Autodesk Inventor part; units mm, degrees
ref_plane "YZ Plane" through (0, 0, 0) normal (1, 0, 0) x (0, 1, 0)
ref_plane "XZ Plane" through (0, 0, 0) normal (0, 1, 0) x (-1, 0, 0)
ref_plane "XY Plane" through (0, 0, 0) normal (0, 0, 1) x (1, 0, 0)
sketch "草圖1" plane through (0, 0, 0) normal (0, 1, 0) x (-1, 0, 0)
  circle A0 centre (0, 0) radius 30
  line L0 (0, -30) -> (-70, -30)
  arc A1 (-70, 30) -> (-70, -30) centre (-70, 0) ccw
  line L1 (0, 30) -> (-70, 30)
  dimension "d0" = 70
  dimension "d1" = 30
  dimension "d2" = 60
extrude "擠出1" add sketch "草圖1" along normal blind 15
sketch "草圖2" plane through (0, 15, 0) normal (0, 1, 0) x (1, 0, 0)
  arc A0 (0, 30) -> (0, -30) centre (0, 0) ccw
  line L0 (0, -30) -> (70, -30)
  arc A1 (70, -30) -> (70, 30) centre (70, 0) ccw
  line L1 (70, 30) -> (0, 30)
  circle A2 centre (0, 0) radius 30
extrude "擠出2" add sketch "草圖2" along normal blind 25 contours A2 A0
sketch "草圖3" plane through (0, 40, 0) normal (0, 1, 0) x (1, 0, 0)
  circle A0 centre (0, 0) radius 16
  dimension "d7" = 32
extrude "擠出3" cut sketch "草圖3" against normal up to next
sketch "草圖4" plane through (0, 40, 0) normal (0, 1, 0) x (1, 0, 0)
  line L0 (-34.5334, 10) -> (33.6388, 10)
  line L1 (33.6388, 10) -> (33.6388, -10)
  line L2 (33.6388, -10) -> (-34.5334, -10)
  line L3 (-34.5334, -10) -> (-34.5334, 10)
  line L4 (-29.5296, 0) -> (41.1192, 0)
  point P0 (0, 0)
  dimension "d10" = 20
extrude "擠出4" cut sketch "草圖4" against normal blind 10
sketch "草圖5" plane through (0, 15, 0) normal (0, 1, 0) x (1, 0, 0)
  line L0 (48.3987, 0) -> (103.2063, 0)
  line L1 (55, 10) -> (80, 10)
  line L2 (55, -10) -> (80, -10)
  arc A0 (80, -10) -> (80, 10) centre (80, 0) ccw
  arc A1 (55, 10) -> (55, -10) centre (55, 0) ccw
  line L3 (0, 0) -> (0, 8.9825) construction
  dimension "d13" = 55
  dimension "d14" = 25
  dimension "d15" = 10
  dimension "d16" = 10
extrude "擠出5" cut sketch "草圖5" against normal blind 5
sketch "草圖6" plane through (0, 10, 0) normal (0, 1, 0) x (1, 0, 0)
  line L0 (55, 5) -> (80, 5)
  arc A0 (55, 5) -> (55, -5) centre (55, 0) ccw
  arc A1 (80, -5) -> (80, 5) centre (80, 0) ccw
  line L1 (55, -5) -> (80, -5)
  line L2 (0, 0) -> (0, 5.5956) construction
  line L3 (0, 0) -> (10.788, 0) construction
  line L4 (0, -30) -> (70, -30)
  dimension "d19" = 55
  dimension "d20" = 25
  dimension "d22" = 5
  dimension "d23" = 5
  dimension "d25" = 30
  dimension "d26" = 0
extrude "擠出6" cut sketch "草圖6" against normal blind 10
properties part number "複習一"
Work out the finished part from the listing and answer in its coordinate system (mm). A direction names the side the tool comes from. Round coordinates to 2 decimals unless told otherwise and drop trailing zeros. Write each loop counter-clockwise with the first axis right and the second up, starting at its lowest first coordinate (ties: lowest second). Pieces come first, ordered by that corner, then holes.
1) A cutting plane is placed at A-A (z = 0). Give the vertices of the cut face in (x, y), plus the area to 4 significant figures.
2) A cutting plane is placed at D-D (y = 20.5). Give the vertices of the cut face in (x, z), plus the area to 3 significant figures.
3) A cutting plane is placed at C-C (z = 13.5). Give the vertices of the cut face in (x, y).
4) The mould has two halves that part along Z. Classify faces 4 (the cylindrical face through (50, 5, 0)), 5 (the flat face through (36, 0, 0)), 6 (the flat face through (35, 7, 30)), 7 (the flat face through (-20, 35, -10)): pulls with the +Z half, pulls with the -Z half, needs draft (parallel to the pull), parting line crosses it, or undercut.
5) Given pin 1 Ø10 at (y, z) = (31, -10) entering from -X; pin 2 Ø3 at (x, y) = (24, 33.5) entering from +Z; pin 3 Ø5 at (x, y) = (-23.5, 33.5) entering from +Z; pin 4 Ø14 at (x, z) = (-19.5, 4) entering from +Y, each flat-ended and moving along its own axis, determine where each tip first touches the part or whether it passes through.
6) A tool of negligible diameter and unlimited length cuts with its end or side. For faces 1 (the cylindrical face through (85, 5, 0)), 2 (the flat face through (20, 35, -10)), 3 (the cylindrical face through (45, 13, 0)), from which of +Z, -Z, +X, -X, +Y, -Y can it reach the whole face along a straight path? Write none if from no direction.
7) Straight lines are drawn through the part: line 1 (X direction, y = 8, z = 0); line 2 (Z direction, x = 0, y = 19); line 3 (Z direction, x = 70.5, y = 7). For each, find the intervals that lie inside material, in ascending order.
8) A cutting plane is placed at B-B (y = 6). Give the vertices of the cut face in (x, z), plus the area to 3 significant figures.
Completed:
1. outline: (-30, 0) - (-16, 0) - (-16, 30) - (-30, 30) - close; (16, 0) - (50, 0) - (50, 10) - (45, 10) - (45, 15) - (30, 15) - (30, 30) - (16, 30) - close; (85, 0) - (100, 0) - (100, 15) - (90, 15) - (90, 10) - (85, 10) - close
1. area: 1,315 mm2
2. outline: circle Ø60 at (0, 0); hole circle Ø32 at (0, 0)
2. area: 2,020 mm2
3. outline: (-26.79, 0) - (-8.59, 0) - (-8.59, 40) - (-26.79, 40) - close; (8.59, 0) - (96.79, 0) - (96.79, 15) - (26.79, 15) - (26.79, 40) - (8.59, 40) - close
4. face 4: undercut
4. face 5: needs draft
4. face 6: pulls with the +Z half
4. face 7: undercut
5. pin 1: stops at x = -29.56
5. pin 2: stops at z = 19.84
5. pin 3: stops at z = 21.42
5. pin 4: stops at y = 40
6. face 1: +Y, -Y
6. face 2: +X, -X, +Y
6. face 3: +Y
7. line 1: x = -30 to -16, 16 to 50, 85 to 100
7. line 2: z = -30 to -16, 16 to 30
7. line 3: z = -30 to -5, 5 to 30
8. outline: (0, -30) - (70, -30) arc R30 ccw to (70, 30) - (0, 30) arc R30 ccw to start; hole circle Ø32 at (0, 0); hole (55, -5) - (80, -5) arc R5 ccw to (80, 5) - (55, 5) arc R5 ccw to start
8. area: 5,890 mm2
